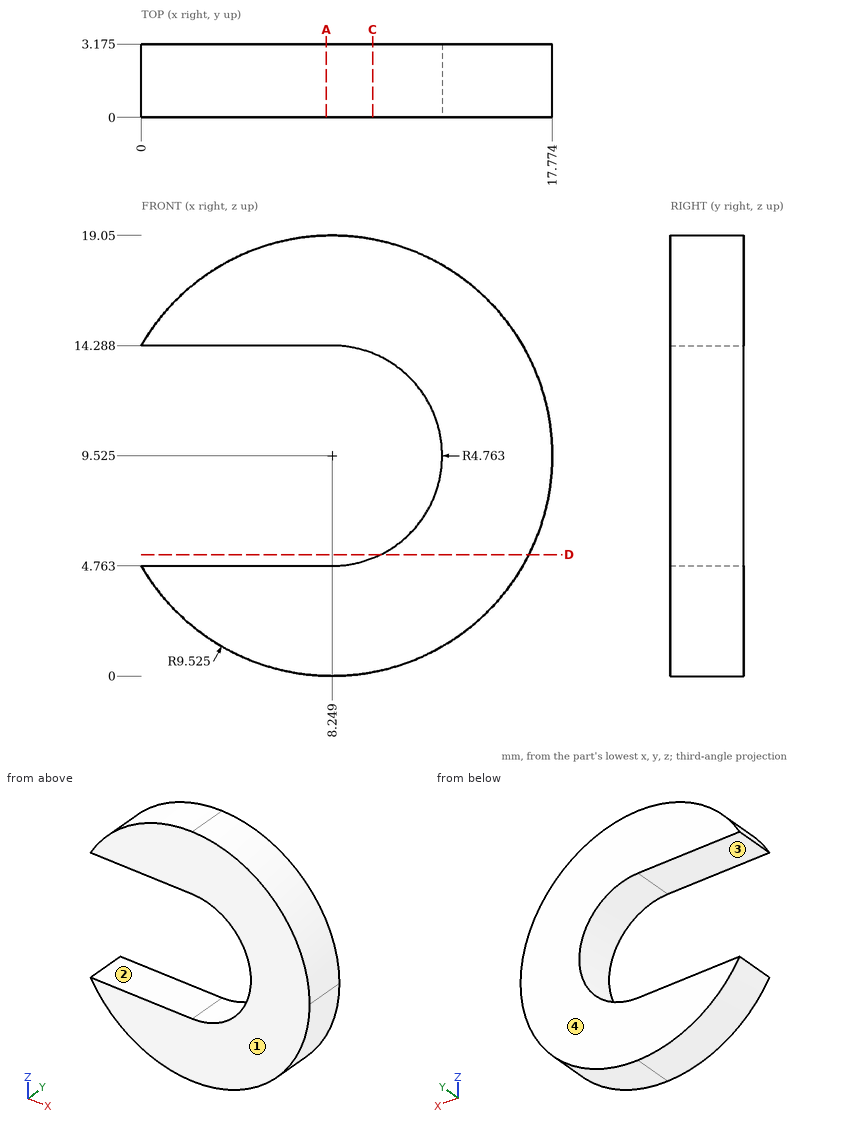
Verification items for this drawing (mm, ordinates from the low corner). A direction names the side the tool comes from. Give positions to 0.01 mm unless a question says otherwise; leave off trailing zeros. Order: outer loops, then holes, each group sorted by start corner. A loop starts at its lowest first (then second) coordinate and runs counter-clockwise, first axis right, second up.
1) Material ranges on probe 1 along Z at (x, y) = (11, 0.95) (1 decimal); probe 2 along Z at (x, y) = (2.5, 1.45) (1 decimal); probe 3 along X at (y, z) = (0.55, 5.5) (1 decimal), recorded low to high.
Results are:
probe 1: z = 0.4 to 5.6, 13.4 to 18.6
probe 2: z = 1.9 to 4.8, 14.3 to 17.1
probe 3: x = 10.8 to 16.9
2) Draft check along Z on the marked faces 1 and 2. Enter one of: released by +Z, released by -Z, zero draft, split by the parting line, or undercut.
Results are:
face 1: zero draft
face 2: undercut
3) Cross-section at D-D (z = 5.25). Record the boundary of the cut face in (x, y) (1 decimal).
Results are:
outline: (10.3, 0) - (16.8, 0) - (16.8, 3.2) - (10.3, 3.2) - close
4) Gauge pin test, flat ends, axial feed: pin 1 (1.6 mm diameter, centred on x = 4.5, y = 1, fed in from -Z); pin 2 (2 mm diameter, centred on x = 11.5, z = 9, fed in from +Y); pin 3 (1 mm diameter, centred on x = 4.5, y = 1.5, fed in from +Z). Record the tip position at first contact, or that the pin passes through.
Results are:
pin 1: stops at z = 0.47
pin 2: passes through
pin 3: stops at z = 18.48
5) Cross-section at C-C (x = 10). Record the boundary of the cut face in (y, z) (1 decimal).
Results are:
outline: (0, 0.2) - (3.2, 0.2) - (3.2, 5.1) - (0, 5.1) - close; (0, 14) - (3.2, 14) - (3.2, 18.9) - (0, 18.9) - close
6) Cross-section at A-A (x = 8). Record the boundary of the cut face in (y, z) (1 decimal).
Results are:
outline: (0, 0) - (3.2, 0) - (3.2, 4.8) - (0, 4.8) - close; (0, 14.3) - (3.2, 14.3) - (3.2, 19) - (0, 19) - close
7) Tool access check on the marked faces 3 and 4. Record the directions out of +Z, -Z, +X, -X, +Y, -Y that give a thin tool (end or side, any length) a straight path to the whole face; none if there is none.
Results are:
face 3: -X, +Y, -Y
face 4: +Z, -Z, +X, -X, +Y
